Design review of the part built by this model. Coordinates are the model's own, in mm. Coordinates: 2 decimals unless noted, no trailing zeros. Loops run counter-clockwise (first coordinate to the right, second up) from the corner with the lowest first, then second, coordinate; pieces in that order, holes last. Notation, with made-up numbers: M 37,85.5 L 85,85.5 A29 ccw 85,118.5 Z; hole C 83,17.25 d5. An arc over 180 degrees is marked long. One line per item, written item: value.
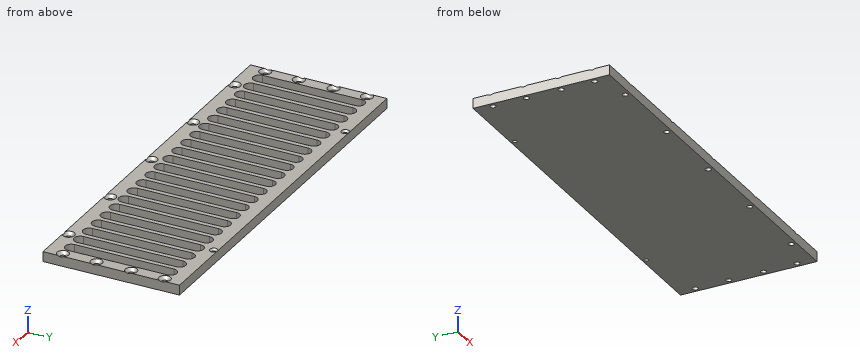
```python
from build123d import *

# Parameters (mm, degrees)
SKETCH1_W                                       = 320
SKETCH1_H                                       = 110
EXTRUDE1_DEPTH                                  = 8
SKETCH2_R                                       = 1.75
CUT_EXTRUDE1_DEPTH                              = 170.378274876
CUT_EXTRUDE2_DEPTH                              = 6
SKETCH6_R                                       = 2.25
CUT_EXTRUDE3_DEPTH                              = 10
SKETCH9_R                                       = 1.5
CUT_EXTRUDE4_DEPTH                              = 10
CSK_FOR_M4_FLAT_HEAD_MACHINE_SCREW1_D           = 4.5
CSK_FOR_M4_FLAT_HEAD_MACHINE_SCREW1_CSINK_D     = 9.4
CSK_FOR_M4_FLAT_HEAD_MACHINE_SCREW1_CSINK_ANGLE = 90
CSK_FOR_M3_FLAT_HEAD_MACHINE_SCREW1_D           = 3.4
CSK_FOR_M3_FLAT_HEAD_MACHINE_SCREW1_CSINK_D     = 6.3
CSK_FOR_M3_FLAT_HEAD_MACHINE_SCREW1_CSINK_ANGLE = 90


with BuildPart() as part:
    # Sketch1 → Extrude1 (new body)
    with BuildSketch(Plane.XY):
        Rectangle(SKETCH1_W, SKETCH1_H)
    extrude(amount=EXTRUDE1_DEPTH)

    # Sketch2 → Cut-Extrude1 (cut, through all)
    with BuildSketch(Plane.XY.offset(8)):
        with Locations((156, 41)):
            Circle(SKETCH2_R)
        with Locations((156, 14)):
            Circle(SKETCH2_R)
        with Locations(Location((156, -14, 0), (0, 0, 180))):
            Circle(SKETCH2_R)
        with Locations(Location((156, -41, 0), (0, 0, 180))):
            Circle(SKETCH2_R)
        with Locations((-156, -41)):
            Circle(SKETCH2_R)
        with Locations((-156, -14)):
            Circle(SKETCH2_R)
        with Locations(Location((-156, 41, 0), (0, 0, 180))):
            Circle(SKETCH2_R)
        with Locations(Location((-156, 14, 0), (0, 0, 180))):
            Circle(SKETCH2_R)
    extrude(amount=-CUT_EXTRUDE1_DEPTH, mode=Mode.SUBTRACT)

    # Sketch5 → Cut-Extrude2 (cut)
    with BuildSketch(Plane.XY.offset(8)):
        with BuildLine():
            Line((150, 40), (150, -40))
            ThreePointArc((150, -40), (145, -45), (140, -40))
            Line((140, -40), (140, 40))
            ThreePointArc((140, 40), (145, 45), (150, 40))
        make_face()
        with BuildLine():
            Line((136.19047619, 40), (136.19047619, -40))
            ThreePointArc((136.19047619, -40), (131.19047619, -45), (126.19047619, -40))
            Line((126.19047619, -40), (126.19047619, 40))
            ThreePointArc((126.19047619, 40), (131.19047619, 45), (136.19047619, 40))
        make_face()
        with BuildLine():
            Line((122.380952381, 40), (122.380952381, -40))
            ThreePointArc((122.380952381, -40), (117.380952381, -45), (112.380952381, -40))
            Line((112.380952381, -40), (112.380952381, 40))
            ThreePointArc((112.380952381, 40), (117.380952381, 45), (122.380952381, 40))
        make_face()
        with BuildLine():
            Line((108.571428571, 40), (108.571428571, -40))
            ThreePointArc((108.571428571, -40), (103.571428571, -45), (98.571428571, -40))
            Line((98.571428571, -40), (98.571428571, 40))
            ThreePointArc((98.571428571, 40), (103.571428571, 45), (108.571428571, 40))
        make_face()
        with BuildLine():
            Line((94.761904762, 40), (94.761904762, -40))
            ThreePointArc((94.761904762, -40), (89.761904762, -45), (84.761904762, -40))
            Line((84.761904762, -40), (84.761904762, 40))
            ThreePointArc((84.761904762, 40), (89.761904762, 45), (94.761904762, 40))
        make_face()
        with BuildLine():
            Line((80.952380952, 40), (80.952380952, -40))
            ThreePointArc((80.952380952, -40), (75.952380952, -45), (70.952380952, -40))
            Line((70.952380952, -40), (70.952380952, 40))
            ThreePointArc((70.952380952, 40), (75.952380952, 45), (80.952380952, 40))
        make_face()
        with BuildLine():
            Line((67.142857143, 40), (67.142857143, -40))
            ThreePointArc((67.142857143, -40), (62.142857143, -45), (57.142857143, -40))
            Line((57.142857143, -40), (57.142857143, 40))
            ThreePointArc((57.142857143, 40), (62.142857143, 45), (67.142857143, 40))
        make_face()
        with BuildLine():
            Line((53.333333333, 40), (53.333333333, -40))
            ThreePointArc((53.333333333, -40), (48.333333333, -45), (43.333333333, -40))
            Line((43.333333333, -40), (43.333333333, 40))
            ThreePointArc((43.333333333, 40), (48.333333333, 45), (53.333333333, 40))
        make_face()
        with BuildLine():
            Line((39.523809524, 40), (39.523809524, -40))
            ThreePointArc((39.523809524, -40), (34.523809524, -45), (29.523809524, -40))
            Line((29.523809524, -40), (29.523809524, 40))
            ThreePointArc((29.523809524, 40), (34.523809524, 45), (39.523809524, 40))
        make_face()
        with BuildLine():
            Line((25.714285714, 40), (25.714285714, -40))
            ThreePointArc((25.714285714, -40), (20.714285714, -45), (15.714285714, -40))
            Line((15.714285714, -40), (15.714285714, 40))
            ThreePointArc((15.714285714, 40), (20.714285714, 45), (25.714285714, 40))
        make_face()
        with BuildLine():
            Line((11.904761905, 40), (11.904761905, -40))
            ThreePointArc((11.904761905, -40), (6.904761905, -45), (1.904761905, -40))
            Line((1.904761905, -40), (1.904761905, 40))
            ThreePointArc((1.904761905, 40), (6.904761905, 45), (11.904761905, 40))
        make_face()
        with BuildLine():
            Line((-1.904761905, 40), (-1.904761905, -40))
            ThreePointArc((-1.904761905, -40), (-6.904761905, -45), (-11.904761905, -40))
            Line((-11.904761905, -40), (-11.904761905, 40))
            ThreePointArc((-11.904761905, 40), (-6.904761905, 45), (-1.904761905, 40))
        make_face()
        with BuildLine():
            Line((-15.714285714, 40), (-15.714285714, -40))
            ThreePointArc((-15.714285714, -40), (-20.714285714, -45), (-25.714285714, -40))
            Line((-25.714285714, -40), (-25.714285714, 40))
            ThreePointArc((-25.714285714, 40), (-20.714285714, 45), (-15.714285714, 40))
        make_face()
        with BuildLine():
            Line((-29.523809524, 40), (-29.523809524, -40))
            ThreePointArc((-29.523809524, -40), (-34.523809524, -45), (-39.523809524, -40))
            Line((-39.523809524, -40), (-39.523809524, 40))
            ThreePointArc((-39.523809524, 40), (-34.523809524, 45), (-29.523809524, 40))
        make_face()
        with BuildLine():
            Line((-43.333333333, 40), (-43.333333333, -40))
            ThreePointArc((-43.333333333, -40), (-48.333333333, -45), (-53.333333333, -40))
            Line((-53.333333333, -40), (-53.333333333, 40))
            ThreePointArc((-53.333333333, 40), (-48.333333333, 45), (-43.333333333, 40))
        make_face()
        with BuildLine():
            Line((-57.142857143, 40), (-57.142857143, -40))
            ThreePointArc((-57.142857143, -40), (-62.142857143, -45), (-67.142857143, -40))
            Line((-67.142857143, -40), (-67.142857143, 40))
            ThreePointArc((-67.142857143, 40), (-62.142857143, 45), (-57.142857143, 40))
        make_face()
        with BuildLine():
            Line((-70.952380952, 40), (-70.952380952, -40))
            ThreePointArc((-70.952380952, -40), (-75.952380952, -45), (-80.952380952, -40))
            Line((-80.952380952, -40), (-80.952380952, 40))
            ThreePointArc((-80.952380952, 40), (-75.952380952, 45), (-70.952380952, 40))
        make_face()
        with BuildLine():
            Line((-84.761904762, 40), (-84.761904762, -40))
            ThreePointArc((-84.761904762, -40), (-89.761904762, -45), (-94.761904762, -40))
            Line((-94.761904762, -40), (-94.761904762, 40))
            ThreePointArc((-94.761904762, 40), (-89.761904762, 45), (-84.761904762, 40))
        make_face()
        with BuildLine():
            Line((-98.571428571, 40), (-98.571428571, -40))
            ThreePointArc((-98.571428571, -40), (-103.571428571, -45), (-108.571428571, -40))
            Line((-108.571428571, -40), (-108.571428571, 40))
            ThreePointArc((-108.571428571, 40), (-103.571428571, 45), (-98.571428571, 40))
        make_face()
        with BuildLine():
            Line((-112.380952381, 40), (-112.380952381, -40))
            ThreePointArc((-112.380952381, -40), (-117.380952381, -45), (-122.380952381, -40))
            Line((-122.380952381, -40), (-122.380952381, 40))
            ThreePointArc((-122.380952381, 40), (-117.380952381, 45), (-112.380952381, 40))
        make_face()
        with BuildLine():
            Line((-126.19047619, 40), (-126.19047619, -40))
            ThreePointArc((-126.19047619, -40), (-131.19047619, -45), (-136.19047619, -40))
            Line((-136.19047619, -40), (-136.19047619, 40))
            ThreePointArc((-136.19047619, 40), (-131.19047619, 45), (-126.19047619, 40))
        make_face()
        with BuildLine():
            Line((-140, 40), (-140, -40))
            ThreePointArc((-140, -40), (-145, -45), (-150, -40))
            Line((-150, -40), (-150, 40))
            ThreePointArc((-150, 40), (-145, 45), (-140, 40))
        make_face()
    extrude(amount=-CUT_EXTRUDE2_DEPTH, mode=Mode.SUBTRACT)

    # Sketch6 → Cut-Extrude3 (cut)
    with BuildSketch(Plane.XY.offset(8)):
        with Locations((-64, -51)):
            Circle(SKETCH6_R)
        with Locations((0, -51)):
            Circle(SKETCH6_R)
        with Locations((64, -51)):
            Circle(SKETCH6_R)
        with Locations((-128, -51)):
            Circle(SKETCH6_R)
        with Locations((128, -51)):
            Circle(SKETCH6_R)
    extrude(amount=-CUT_EXTRUDE3_DEPTH, mode=Mode.SUBTRACT)

    # Sketch9 → Cut-Extrude4 (cut)
    with BuildSketch(Plane.XY.offset(8)):
        with Locations((101.5, 52)):
            Circle(SKETCH9_R)
        with Locations((-101.5, 52)):
            Circle(SKETCH9_R)
    extrude(amount=-CUT_EXTRUDE4_DEPTH, mode=Mode.SUBTRACT)

    # CSK for M4 Flat Head Machine Screw1 (through all)
    with Locations(Plane.XY.offset(8)):
        with Locations((156, 41), (156, 14), (156, -14), (156, -41), (-156, -41), (-156, -14), (-156, 14), (-156, 41), (-128, -51), (-64, -51), (0, -51), (64, -51), (128, -51)):
            CounterSinkHole(CSK_FOR_M4_FLAT_HEAD_MACHINE_SCREW1_D / 2, CSK_FOR_M4_FLAT_HEAD_MACHINE_SCREW1_CSINK_D / 2, counter_sink_angle=CSK_FOR_M4_FLAT_HEAD_MACHINE_SCREW1_CSINK_ANGLE)

    # CSK for M3 Flat Head Machine Screw1 (through all)
    with Locations(Plane.XY.offset(8)):
        with Locations((-101.5, 52), (101.5, 52)):
            CounterSinkHole(CSK_FOR_M3_FLAT_HEAD_MACHINE_SCREW1_D / 2, CSK_FOR_M3_FLAT_HEAD_MACHINE_SCREW1_CSINK_D / 2, counter_sink_angle=CSK_FOR_M3_FLAT_HEAD_MACHINE_SCREW1_CSINK_ANGLE)


solid = part.part
```
(1) To check wall thickness, follow line 1 along X through (y, z) = (-14, 1.3); line 2 along X through (y, z) = (-51, 1.9); line 3 along Y through (x, z) = (156, 1.25). State the ranges of each line that lie inside material, in increasing order. Write a range as [from, to].
Reply:
line 1: x = [-160, -158.25], [-153.75, 153.75], [158.25, 160]
line 2: x = [-160, -130.25], [-125.75, -66.25], [-61.75, -2.25], [2.25, 61.75], [66.25, 125.75], [130.25, 160]
line 3: y = [-55, -43.25], [-38.75, -16.25], [-11.75, 11.75], [16.25, 38.75], [43.25, 55]
(2) We need section B-B on x = 18.5. State the section outline as (y, z) points, then the cut area to 3 significant figures.
Reply:
outline: M -55,0 L 55,0 L 55,8 L 44.48,8 L 44.48,2 L -44.48,2 L -44.48,8 L -55,8 Z
area: 346 mm2
(3) We need section A-A on x = -145. State the section outline as (y, z) points, then the cut area to 3 significant figures.
Reply:
outline: M -55,0 L 55,0 L 55,8 L 45,8 L 45,2 L -45,2 L -45,8 L -55,8 Z
area: 340 mm2
(4) Insertion check: pin 1 (5 mm diameter, centred on x = 156, y = -41, fed in from +Z); pin 2 (6 mm diameter, centred on x = 156, y = 41, fed in from +Z); pin 3 (7 mm diameter, centred on x = -64, y = -51, fed in from +Z). Each pin has a flat end and moves straight along its axis. Give the tip position at first contact, or say it passes through.
Reply:
pin 1: stops at z = 5.8
pin 2: stops at z = 6.3
pin 3: stops at z = 6.8
